For this review, take the finished solid that the model builds, in its own axes (mm). A direction names the side the tool comes from. Coordinates: 2 decimals unless noted, no trailing zeros. Write each loop counter-clockwise with the first axis right and the second up, starting at its lowest first coordinate (ties: lowest second). Pieces come first, ordered by that corner, then holes. Notation, with made-up numbers: M 65,53 L 79,53 A33 ccw 79,91 Z; hole C 54.5,-9 d9. An arc over 180 degrees is marked long. Return JSON: item names as keys, results as strings.
```python
from build123d import *

# Parameters (mm, degrees)
BOSS_EXTRUDE1_DEPTH     = 2.5
SKETCH3_W               = 16
SKETCH3_H               = 63
BOSS_EXTRUDE2_DEPTH     = 15
SKETCH2_R               = 1.5
CUT_EXTRUDE1_DEPTH      = 3.5
CUT_EXTRUDE1_DEPTH_BACK = 17
CUT_EXTRUDE2_DEPTH      = 1
CUT_EXTRUDE2_TAPER      = 45
SKETCH5_W               = 11.73250701
SKETCH5_H               = 7.616061756
CUT_EXTRUDE3_DEPTH      = 1


with BuildPart() as part:
    # Sketch1 → Boss-Extrude1 (new body)
    with BuildSketch(Plane.XY):
        with BuildLine():
            Line((-12, 35), (12, 35))
            ThreePointArc((12, 35), (14.474873734, 33.974873734), (15.5, 31.5))
            Line((15.5, 31.5), (15.5, -31.5))
            ThreePointArc((15.5, -31.5), (14.474873734, -33.974873734), (12, -35))
            Line((12, -35), (-12, -35))
            ThreePointArc((-12, -35), (-14.474873734, -33.974873734), (-15.5, -31.5))
            Line((-15.5, -31.5), (-15.5, 31.5))
            ThreePointArc((-15.5, 31.5), (-14.474873734, 33.974873734), (-12, 35))
        make_face()
    extrude(amount=BOSS_EXTRUDE1_DEPTH)

    # Sketch3 → Boss-Extrude2 (add, symmetric)
    with BuildSketch(Plane(origin=(0, 0, 0), x_dir=(0, 0, -1), z_dir=(1, 0, 0))):
        with Locations((8, 0)):
            Rectangle(SKETCH3_W, SKETCH3_H)
    extrude(amount=BOSS_EXTRUDE2_DEPTH, both=True)

    # Sketch2 → Cut-Extrude1 (cut, two sides)
    with BuildSketch(Plane.XY) as cut_extrude1_sk:
        with Locations((-12, -31.5)):
            Circle(SKETCH2_R)
        with Locations((12, -31.5)):
            Circle(SKETCH2_R)
        with Locations((12, 31.5)):
            Circle(SKETCH2_R)
        with Locations((-12, 31.5)):
            Circle(SKETCH2_R)
    extrude(amount=CUT_EXTRUDE1_DEPTH, mode=Mode.SUBTRACT)
    extrude(cut_extrude1_sk.sketch, amount=-CUT_EXTRUDE1_DEPTH_BACK, mode=Mode.SUBTRACT)

    # Sketch4 → Cut-Extrude2 (cut)
    with BuildSketch(Plane.XY.offset(2.5)):
        with BuildLine():
            ThreePointArc((13.5, 1.5), (0, 15), (-13.5, 1.5))
            Line((-13.5, 1.5), (-13.5, -9.5))
            ThreePointArc((-13.5, -9.5), (0, -23), (13.5, -9.5))
            Line((13.5, -9.5), (13.5, 1.5))
        make_face()
    extrude(amount=-CUT_EXTRUDE2_DEPTH, taper=CUT_EXTRUDE2_TAPER, mode=Mode.SUBTRACT)

    # Sketch5 → Cut-Extrude3 (cut)
    with BuildSketch(Plane(origin=(0, 31.5, 0), x_dir=(1, 0, 0), z_dir=(0, 1, 0))):
        with Locations((0, 8)):
            Rectangle(SKETCH5_W, SKETCH5_H)
    extrude(amount=-CUT_EXTRUDE3_DEPTH, mode=Mode.SUBTRACT)


solid = part.part
```
1. Wall thickness on L1, parallel to Y at x = 12, z = 0.55; L2, parallel to X at y = -31.5, z = 1.95; L3, parallel to Y at x = -12, z = -13.75: over which ranges is each line inside the solid? List them lowest first. Write a range as from..to.
Checks:
{"L1": "-35..-33, -30..30, 33..35", "L2": "-15.5..-13.5, -10.5..10.5, 13.5..15.5", "L3": "-30..30"}
2. We need section B-B (y = 24.5). State the section outline as (x, z) points.
Checks:
{"outline": "M -15.5,0 L -15,0 L -15,-16 L 15,-16 L 15,0 L 15.5,0 L 15.5,2.5 L -15.5,2.5 Z"}
3. Clearance check with flat-ended pins moving along their axes: pin 1 Ø1.2 at (x, z) = (14, -4.5) entering from -Y; pin 2 Ø0.8 at (y, z) = (31, -7) entering from +X; pin 3 Ø2 at (y, z) = (10, -11) entering from -X. State where each tip first meets the part, or that it passes through.
Checks:
{"pin 1": "y = -31.5", "pin 2": "x = 15", "pin 3": "x = -15"}
4. For faces 1 (the face through (-15, 0, -8)), 2 (the face through (0, 31.5, -13)), 3 (the face through (14, -31.5, -8)), 4 (the face through (0, 30.5, -8)), list the 3-axis set-ups (+Z, -Z, +X, -X, +Y, -Y) from which the entire face can be reached by the end or side of a thin tool; tool diameter is ignored.
Checks:
{"face 1": "-Z, -X, +Y, -Y", "face 2": "-Z, +X, -X, +Y", "face 3": "-Z, +X, -X, -Y", "face 4": "+Y"}
5. We need section C-C (z = 0.75). State the section outline as (x, y) points, plus the area to 3 significant figures.
Checks:
{"outline": "M -15.5,-31.5 A3.5 ccw -12,-35 L 12,-35 A3.5 ccw 15.5,-31.5 L 15.5,31.5 A3.5 ccw 12,35 L -12,35 A3.5 ccw -15.5,31.5 Z; hole C -12,-31.5 d3; hole C -12,31.5 d3; hole C 12,-31.5 d3; hole C 12,31.5 d3", "area": "2,130 mm2"}
6. Draft analysis for pull direction Y (two halves, no side actions). For faces 5 (the face through (15, 0, -8)), 6 (the face through (-0.278, -22.157, 1.66)), 7 (the face through (-14, -31.5, -8)), state which applies: +Y half, -Y half, draft (parallel to the pull), parting line (faces both ways), or undercut.
Checks:
{"face 5": "draft", "face 6": "undercut", "face 7": "-Y half"}
7. We need section A-A (z = -6). State the section outline as (x, y) points, plus the area to 3 significant figures.
Checks:
{"outline": "M -15,-31.5 L -13.5,-31.5 A1.5 cw -10.5,-31.5 L 10.5,-31.5 A1.5 cw 13.5,-31.5 L 15,-31.5 L 15,31.5 L 13.5,31.5 A1.5 cw 10.5,31.5 L 5.87,31.5 L 5.87,30.5 L -5.87,30.5 L -5.87,31.5 L -10.5,31.5 A1.5 cw -13.5,31.5 L -15,31.5 Z", "area": "1,860 mm2"}
8. We need section D-D (y = -4.5). State the section outline as (x, z) points.
Checks:
{"outline": "M -15.5,0 L -15,0 L -15,-16 L 15,-16 L 15,0 L 15.5,0 L 15.5,2.5 L 13.5,2.5 L 12.5,1.5 L -12.5,1.5 L -13.5,2.5 L -15.5,2.5 Z"}
